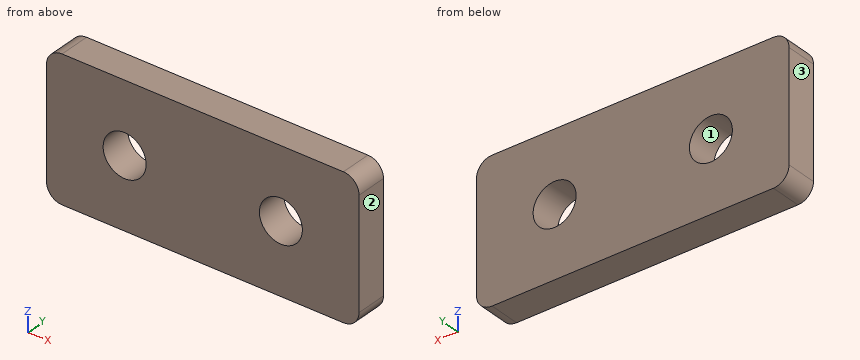
from build123d import *

# Parameters (mm, degrees)
SKETCH_1_W          = 40
SKETCH_1_H          = 18
EXTRUDE_1_DEPTH     = 4
SKETCH_2_R          = 2.75
CUT_EXTRUDE_1_DEPTH = 4
FILLET_1_R          = 2


with BuildPart() as part:
    # 草图1 → 凸台-拉伸1 (new body)
    with BuildSketch(Plane(origin=(0, 0, 0), x_dir=(1, 0, 0), z_dir=(0, 1, 0))):
        Rectangle(SKETCH_1_W, SKETCH_1_H)
    extrude(amount=EXTRUDE_1_DEPTH)

    # 草图2 → 切除-拉伸1 (cut)
    with BuildSketch(Plane(origin=(0, 4, 0), x_dir=(1, 0, 0), z_dir=(0, 1, 0))):
        with Locations(Location((-10, 0, 0), (0, 0, 270))):
            Circle(SKETCH_2_R)
        with Locations(Location((10, 0, 0), (0, 0, 90))):
            Circle(SKETCH_2_R)
    extrude(amount=-CUT_EXTRUDE_1_DEPTH, mode=Mode.SUBTRACT)

    # 圆角1
    fillet_1_edges = [part.edges().sort_by_distance(p)[0] for p in [
        (20, 2, 9),
        (-20, 2, 9),
        (-20, 2, -9),
        (20, 2, -9),
    ]]
    fillet(fillet_1_edges, radius=FILLET_1_R)


solid = part.part
Geometry check sheet. Reference: the model listing, model coordinates, mm. Face numbers are marked on the shaded views. Round coordinates to 2 decimals unless told otherwise and drop trailing zeros. Loops run counter-clockwise (first coordinate to the right, second up) from the corner with the lowest first, then second, coordinate; pieces in that order, holes last.
Item 1: Cross-section at D-D on z = 8.25. Record the boundary of the cut face in (x, y).
Item 2: Cross-section at B-B on y = 3.2. Record the boundary of the cut face in (x, z), then the cut area to 3 significant figures.
Item 3: Thickness scan on line 1 (X direction, y = 1.5, z = 0); line 2 (X direction, y = 1.35, z = -2.25); line 3 (Z direction, x = 10, y = 0.85). Record the ranges inside material, lowest first.
Item 4: Mould release check, pull along X, two halves, no side actions. Record for the marked faces 1, 2 and 3: pulls with the +X half, pulls with the -X half, needs draft (parallel to the pull), parting line crosses it, or undercut.
Item 5: Cross-section at C-C on x = 10. Record the boundary of the cut face in (y, z).
Item 6: Cross-section at A-A on z = 0. Record the boundary of the cut face in (x, y).
Item 7: Gauge pin test, flat end, axial feed: pin 1 (3.5 mm diameter, centred on x = -10, z = 0, fed in from -Y). Record the tip position at first contact, or that the pin passes through.
Answer sheet:
1. outline: (-19.56, 0) - (19.56, 0) - (19.56, 4) - (-19.56, 4) - close
2. outline: (-20, -7) arc R2 ccw to (-18, -9) - (18, -9) arc R2 ccw to (20, -7) - (20, 7) arc R2 ccw to (18, 9) - (-18, 9) arc R2 ccw to (-20, 7) - close; hole circle Ø5.5 at (-10, 0); hole circle Ø5.5 at (10, 0)
2. area: 669 mm2
3. line 1: x = -20 to -12.75, -7.25 to 7.25, 12.75 to 20
3. line 2: x = -20 to -11.58, -8.42 to 8.42, 11.58 to 20
3. line 3: z = -9 to -2.75, 2.75 to 9
4. face 1: undercut
4. face 2: pulls with the +X half
4. face 3: pulls with the -X half
5. outline: (0, -9) - (4, -9) - (4, -2.75) - (0, -2.75) - close; (0, 2.75) - (4, 2.75) - (4, 9) - (0, 9) - close
6. outline: (-20, 0) - (-12.75, 0) - (-12.75, 4) - (-20, 4) - close; (-7.25, 0) - (7.25, 0) - (7.25, 4) - (-7.25, 4) - close; (12.75, 0) - (20, 0) - (20, 4) - (12.75, 4) - close
7. pin 1: passes through
